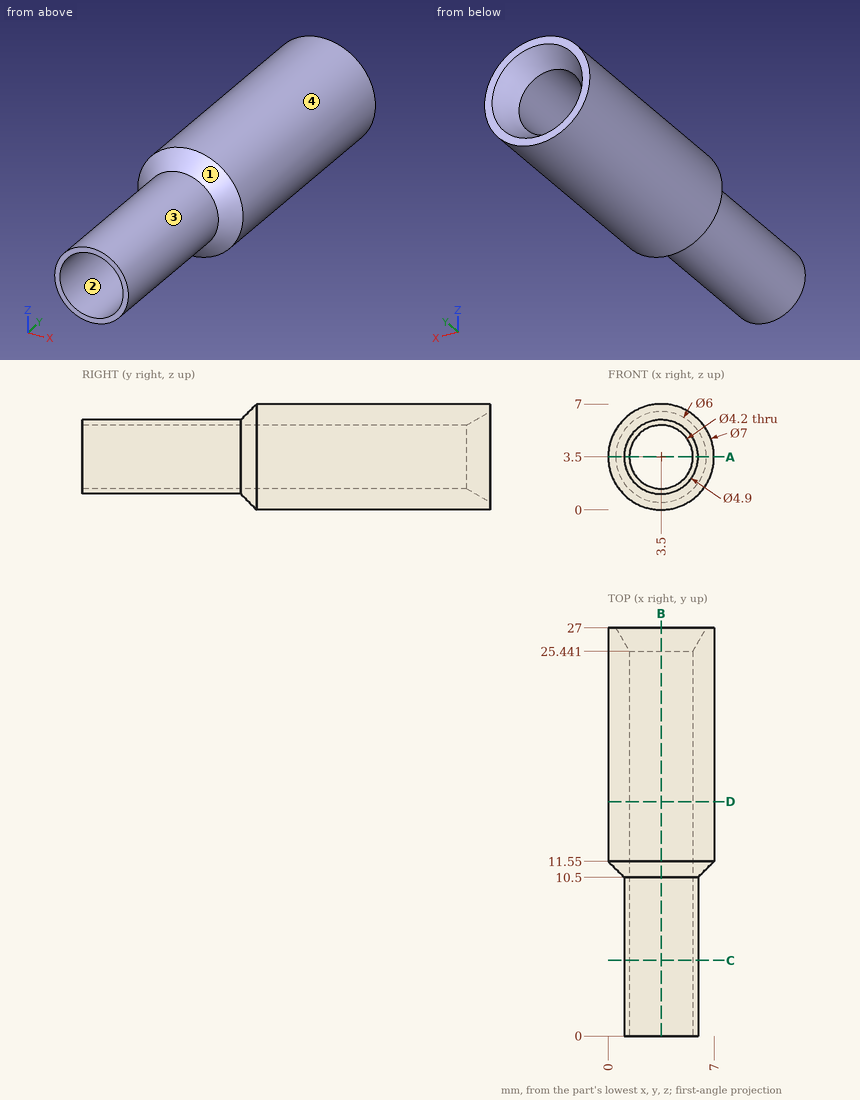
Could you check a few things on this drawing? It's one solid part, dimensions in mm from its lowest x, y, z. A direction names the side the tool comes from. Round coordinates to 2 decimals unless told otherwise and drop trailing zeros. Order: outer loops, then holes, each group sorted by start corner. A loop starts at its lowest first (then second) coordinate and runs counter-clockwise, first axis right, second up.
Q1. Which directions (+Z, -Z, +X, -X, +Y, -Y) give clear straight access to the entire face, cutting with the end or side of a thin tool? Please do the marked faces 3 and 4.
Geometry says:
face 3: -Y
face 4: +Y, -Y
Q2. Thinking about a two-plate mould opening in Z: for the marked faces 1 and 2, which applies, released by +Z, released by -Z, zero draft, split by the parting line, or undercut?
Geometry says:
face 1: split by the parting line
face 2: undercut
Q3. Please list where these lines run through material, in increasing order: probe 1 along Z at (x, y) = (3.5, 15); probe 2 along Z at (x, y) = (3.5, 7.5).
Geometry says:
probe 1: z = 0 to 1.4, 5.6 to 7
probe 2: z = 1.05 to 1.4, 5.6 to 5.95
Q4. Imagine slicing it at C-C, the plane y = 5. List the corners of the cut face in (x, z) for me.
Geometry says:
outline: circle Ø4.9 at (3.5, 3.5); hole circle Ø4.2 at (3.5, 3.5)
Q5. Imagine slicing it at B-B, the plane x = 3.5. List the corners of the cut face in (y, z) for me.
Geometry says:
outline: (0, 1.05) - (10.5, 1.05) - (11.55, 0) - (27, 0) - (27, 0.5) - (25.44, 1.4) - (0, 1.4) - close; (0, 5.6) - (25.44, 5.6) - (27, 6.5) - (27, 7) - (11.55, 7) - (10.5, 5.95) - (0, 5.95) - close
Q6. Imagine slicing it at D-D, the plane y = 15.5. List the corners of the cut face in (x, z) for me, then the cut area to 3 significant figures.
Geometry says:
outline: circle Ø7 at (3.5, 3.5); hole circle Ø4.2 at (3.5, 3.5)
area: 24.6 mm2
Q7. I'm going to push flat-ended pins straight in: P1, Ø1.5, axis at y = 5, z = 6, coming from the +X side (1 decimal); P2, Ø1, axis at y = 7.5, z = 1.5, coming from the -X side; P3, Ø3, axis at y = 12.5, z = 5.5, coming from the -X side; P4, Ø4, axis at x = 3.5, z = 3.5, coming from the -Y side. Where does each tip first touch, or does it pass through?
Geometry says:
P1: stops at x = 5.2
P2: stops at x = 1.56
P3: stops at x = 0.04
P4: passes through
Q8. Imagine slicing it at A-A, the plane z = 3.5. List the corners of the cut face in (x, y) for me.
Geometry says:
outline: (0, 11.55) - (1.05, 10.5) - (1.05, 0) - (1.4, 0) - (1.4, 25.44) - (0.5, 27) - (0, 27) - close; (5.6, 0) - (5.95, 0) - (5.95, 10.5) - (7, 11.55) - (7, 27) - (6.5, 27) - (5.6, 25.44) - close
